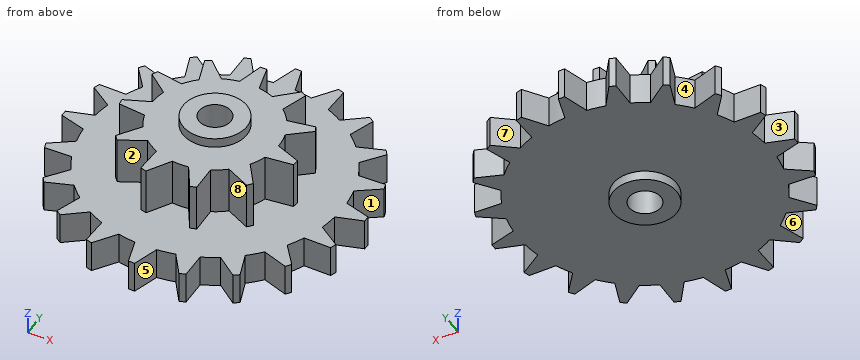
```python
from build123d import *

# Parameters (mm, degrees)
SKETCH1_R                = 40
BOSS_EXTRUDE1_DEPTH      = 10
BOSS_EXTRUDE2_DEPTH      = 10
SKETCH3_R                = 20
BOSS_EXTRUDE3_DEPTH      = 15
BOSS_EXTRUDE4_START      = -15
BOSS_EXTRUDE4_DEPTH      = 15
BOSS_EXTRUDE6_DEPTH      = 3
BOSS_EXTRUDE6_DEPTH_BACK = 28
SKETCH5_R                = 10
SKETCH5_R_2              = 5
CUT_EXTRUDE1_DEPTH       = 74.430239003
CUT_EXTRUDE1_DEPTH_BACK  = 74.430239003
SKETCH6_R                = 5


with BuildPart() as part:
    # Sketch1 → Boss-Extrude1 (new body)
    with BuildSketch(Plane.XY):
        Circle(SKETCH1_R)
    extrude(amount=BOSS_EXTRUDE1_DEPTH)

    # Sketch2 → Boss-Extrude2 (add)
    with BuildSketch(Plane.XY.offset(10)):
        Polygon((-1, 48), (1, 48), (4, 38), (-4, 38), align=None)
        Polygon((7.938419721, 37.376215597), (13.881759214, 45.959729777), (15.783872246, 45.341695788), (15.546871851, 34.904079642), align=None)
        Polygon((19.09977161, 33.093786795), (27.404675116, 39.420600982), (29.022709104, 38.245030478), (25.571907565, 28.391504777), align=None)
        Polygon((28.391504777, 25.571907565), (38.245030478, 29.022709104), (39.420600982, 27.404675116), (33.093786795, 19.09977161), align=None)
        Polygon((34.904079642, 15.546871851), (45.341695788, 15.783872246), (45.959729777, 13.881759214), (37.376215597, 7.938419721), align=None)
        Polygon((38, 4), (48, 1), (48, -1), (38, -4), align=None)
        Polygon((37.376215597, -7.938419721), (45.959729777, -13.881759214), (45.341695788, -15.783872246), (34.904079642, -15.546871851), align=None)
        Polygon((33.093786795, -19.09977161), (39.420600982, -27.404675116), (38.245030478, -29.022709104), (28.391504777, -25.571907565), align=None)
        Polygon((25.571907565, -28.391504777), (29.022709104, -38.245030478), (27.404675116, -39.420600982), (19.09977161, -33.093786795), align=None)
        Polygon((15.546871851, -34.904079642), (15.783872246, -45.341695788), (13.881759214, -45.959729777), (7.938419721, -37.376215597), align=None)
        Polygon((4, -38), (1, -48), (-1, -48), (-4, -38), align=None)
        Polygon((-7.938419721, -37.376215597), (-13.881759214, -45.959729777), (-15.783872246, -45.341695788), (-15.546871851, -34.904079642), align=None)
        Polygon((-19.09977161, -33.093786795), (-27.404675116, -39.420600982), (-29.022709104, -38.245030478), (-25.571907565, -28.391504777), align=None)
        Polygon((-28.391504777, -25.571907565), (-38.245030478, -29.022709104), (-39.420600982, -27.404675116), (-33.093786795, -19.09977161), align=None)
        Polygon((-34.904079642, -15.546871851), (-45.341695788, -15.783872246), (-45.959729777, -13.881759214), (-37.376215597, -7.938419721), align=None)
        Polygon((-38, -4), (-48, -1), (-48, 1), (-38, 4), align=None)
        Polygon((-37.376215597, 7.938419721), (-45.959729777, 13.881759214), (-45.341695788, 15.783872246), (-34.904079642, 15.546871851), align=None)
        Polygon((-33.093786795, 19.09977161), (-39.420600982, 27.404675116), (-38.245030478, 29.022709104), (-28.391504777, 25.571907565), align=None)
        Polygon((-25.571907565, 28.391504777), (-29.022709104, 38.245030478), (-27.404675116, 39.420600982), (-19.09977161, 33.093786795), align=None)
        Polygon((-15.546871851, 34.904079642), (-15.783872246, 45.341695788), (-13.881759214, 45.959729777), (-7.938419721, 37.376215597), align=None)
    extrude(amount=-BOSS_EXTRUDE2_DEPTH)

    # Sketch3 → Boss-Extrude3 (add)
    with BuildSketch(Plane.XY.offset(10)):
        Circle(SKETCH3_R)
    extrude(amount=BOSS_EXTRUDE3_DEPTH)

    # Sketch4 → Boss-Extrude4 (add)
    with BuildSketch(Plane.XY.offset(25).offset(BOSS_EXTRUDE4_START)):
        with BuildLine():
            ThreePointArc((-13.298978315, 14.937776802), (-10.804143602, 16.830641136), (-8.044414634, 18.310854518))
            Line((-8.044414634, 18.310854518), (-14.296689356, 24.095739737))
            Line((-14.296689356, 24.095739737), (-15.979196422, 23.014458102))
            Line((-15.979196422, 23.014458102), (-13.298978315, 14.937776802))
        make_face()
        with BuildLine():
            Line((1, 28), (-1, 28))
            Line((-1, 28), (-3.11184063, 19.756428015))
            ThreePointArc((-3.11184063, 19.756428015), (-1.560679292, 19.939014021), (0, 20))
            ThreePointArc((0, 20), (1.570955262, 19.93820703), (3.132203125, 19.753209957))
            Line((3.132203125, 19.753209957), (1, 28))
        make_face()
        with BuildLine():
            Line((14.296689356, 24.095739737), (8.063284469, 18.302552925))
            ThreePointArc((8.063284469, 18.302552925), (10.821486224, 16.819495709), (13.314368522, 14.924060803))
            Line((13.314368522, 14.924060803), (15.979196422, 23.014458102))
            Line((15.979196422, 23.014458102), (14.296689356, 24.095739737))
        make_face()
        with BuildLine():
            Line((25.054280857, 12.541252359), (16.67837372, 11.037746602))
            ThreePointArc((16.67837372, 11.037746602), (18.196919426, 8.298923027), (19.269315989, 5.356627793))
            Line((19.269315989, 5.356627793), (25.885110883, 10.721988369))
            Line((25.885110883, 10.721988369), (25.054280857, 12.541252359))
        make_face()
        with BuildLine():
            Line((27.857315211, -2.99499403), (19.99819716, 0.268533721))
            ThreePointArc((19.99819716, 0.268533721), (19.999549285, 0.134269886), (20, 0))
            ThreePointArc((20, 0), (19.775336098, -2.989328052), (19.10639178, -5.911496693))
            Line((19.10639178, -5.911496693), (27.572685534, -4.974636914))
            Line((27.572685534, -4.974636914), (27.857315211, -2.99499403))
        make_face()
        with BuildLine():
            ThreePointArc((-19.263784352, 5.376486999), (-18.188355556, 8.317675286), (-16.666987586, 11.054932149))
            Line((-16.666987586, 11.054932149), (-25.054280857, 12.541252359))
            Line((-25.054280857, 12.541252359), (-25.885110883, 10.721988369))
            Line((-25.885110883, 10.721988369), (-19.263784352, 5.376486999))
        make_face()
        with BuildLine():
            ThreePointArc((-19.112474968, -5.891799437), (-19.797893134, -2.836093696), (-19.997909742, 0.289146933))
            Line((-19.997909742, 0.289146933), (-27.857315211, -2.99499403))
            Line((-27.857315211, -2.99499403), (-27.572685534, -4.974636914))
            Line((-27.572685534, -4.974636914), (-19.112474968, -5.891799437))
        make_face()
        with BuildLine():
            ThreePointArc((-12.893089824, -15.289481181), (-15.121739527, -13.089422969), (-16.979636854, -10.568440392))
            Line((-16.979636854, -10.568440392), (-21.815848816, -17.580350976))
            Line((-21.815848816, -17.580350976), (-20.506127348, -19.091850125))
            Line((-20.506127348, -19.091850125), (-12.893089824, -15.289481181))
        make_face()
        with BuildLine():
            ThreePointArc((-2.580239759, -19.832860681), (-5.644540466, -19.186952935), (-8.570449237, -18.070622565))
            Line((-8.570449237, -18.070622565), (-8.848004565, -26.584070704))
            Line((-8.848004565, -26.584070704), (-6.929018618, -27.147535818))
            Line((-6.929018618, -27.147535818), (-2.580239759, -19.832860681))
        make_face()
        with BuildLine():
            Line((8.848004565, -26.584070704), (8.551818198, -18.079447047))
            ThreePointArc((8.551818198, -18.079447047), (5.624760311, -19.192760912), (2.559795457, -19.835509754))
            Line((2.559795457, -19.835509754), (6.929018618, -27.147535818))
            Line((6.929018618, -27.147535818), (8.848004565, -26.584070704))
        make_face()
        with BuildLine():
            Line((21.815848816, -17.580350976), (16.968734301, -10.585936718))
            ThreePointArc((16.968734301, -10.585936718), (15.108239432, -13.10500291), (12.87732318, -15.302762748))
            Line((12.87732318, -15.302762748), (20.506127348, -19.091850125))
            Line((20.506127348, -19.091850125), (21.815848816, -17.580350976))
        make_face()
    extrude(amount=BOSS_EXTRUDE4_DEPTH)

    # Sketch5 → Boss-Extrude6 (add, two sides: drawn at the far end of the back side and taken through both)
    with BuildSketch(Plane.XY.offset(25).offset(-BOSS_EXTRUDE6_DEPTH_BACK)):
        Circle(SKETCH5_R)
        Circle(SKETCH5_R_2, mode=Mode.SUBTRACT)
    extrude(amount=BOSS_EXTRUDE6_DEPTH + BOSS_EXTRUDE6_DEPTH_BACK)

    # Sketch6 → Cut-Extrude1 (cut, two sides: drawn at the far end of the back side and taken through both)
    with BuildSketch(Plane.XY.offset(25).offset(-CUT_EXTRUDE1_DEPTH_BACK)):
        Circle(SKETCH6_R)
    extrude(amount=CUT_EXTRUDE1_DEPTH + CUT_EXTRUDE1_DEPTH_BACK, mode=Mode.SUBTRACT)


solid = part.part
```
Input: part model. Units: mm. Frame: model coordinates. Face numbers are marked on the shaded views. A direction names the side the tool comes from. Coordinates: 2 decimals unless noted, no trailing zeros. Write each loop counter-clockwise with the first axis right and the second up, starting at its lowest first coordinate (ties: lowest second). Pieces come first, ordered by that corner, then holes. Notation, with made-up numbers: (-26, -18) -> (18, -18) arc R5 cw to (18, -14) -> close; hole circle Ø2 at (26.5, 12.25). An arc over 180 degrees is marked (long way). Write each question's results on one line, items separated by ' | '.
Item 1: Mould query, pull axis Y, two halves, no side actions, for the marked faces 6, 7 and 8. Classes: +Y half, -Y half, draft (parallel to the pull), parting line (faces both ways), or undercut.
Conclusion:
face 6: undercut | face 7: +Y half | face 8: -Y half
Item 2: Pin query (flat end, axial travel): pin 1 Ø4 at (x, y) = (20, -5.5) entering from -Z; pin 2 Ø1 at (y, z) = (12, 1.5) entering from -X; pin 3 Ø8 at (x, y) = (0, 0) entering from -Z; pin 4 Ø1 at (x, z) = (6.5, 1.5) entering from +Y. Return the tip coordinate at first contact, or that it passes through.
Conclusion:
pin 1: stops at z = 0 | pin 2: stops at x = -43.96 | pin 3: passes through | pin 4: stops at y = 39.55
Item 3: Section query A-A on y = -32. Return loops of the section in (x, z), plus the area to 3 significant figures.
Conclusion:
outline: (-26.84, 0) -> (26.84, 0) -> (26.84, 10) -> (-26.84, 10) -> close | area: 537 mm^2
Item 4: Material intervals for probe 1 along Y at (x, z) = (0, 11); probe 2 along X at (y, z) = (42.5, 1.5); probe 3 along Y at (x, z) = (0, 9), sorted ascending.
Conclusion:
probe 1: y = -20 to -5, 5 to 28 | probe 2: x = -15.72 to -11.49, -2.65 to 2.65, 11.49 to 15.72 | probe 3: y = -48 to -5, 5 to 48
Item 5: Set-up query: the marked faces 1, 2, 3, 4 and 5. Return all of +Z, -Z, +X, -X, +Y, -Y with unobstructed straight access to the full face (end or side cutting, diameter ignored); none if empty.
Conclusion:
face 1: +Z, -Z, +X | face 2: +Z, -Y | face 3: +Z, -Z, -X | face 4: +Z, -Z | face 5: +Z, -Z, -Y
